Build history of the part. All positions in model axes, mm. Face numbers are marked on the shaded views. A direction names the side the tool comes from. Give positions to 0.01 mm unless a question says otherwise; leave off trailing zeros. Write each loop counter-clockwise with the first axis right and the second up, starting at its lowest first coordinate (ties: lowest second). Pieces come first, ordered by that corner, then holes. Notation, with made-up numbers: (-34, 54) -> (10, 54) arc R20 ccw to (10, 87) -> close; hole circle Ø7 at (1, 65.5). An arc over 180 degrees is marked (long way). Put each result on its own line as item: value. Start each with the question number.
Item 1: Drill centre lines: line 1 along Y through (x, z) = (0, -5.5); line 2 along Y through (x, z) = (10, -6.75); line 3 along Y through (x, z) = (-10, -10.25). Where is each one in solid material? Low to high.
Item 2: Slice it at B-B, the plane z = -1.25. Give the number of separate pieces and of enclosed holes in the cut face, plus the area to 3 significant figures.
Item 3: Tool access for the marked faces 1 and 2: list every direction of +Z, -Z, +X, -X, +Y, -Y with a clear straight run to the whole face (end or side of a thin tool).
Item 4: Flat gauge pins, fed straight in: pin 1 Ø3 at (x, z) = (-11.5, -2.5) entering from -Y; pin 2 Ø6 at (x, y) = (-2, 22) entering from +Z; pin 3 Ø5 at (y, z) = (22.5, -4) entering from -X. Where does each tip first touch, or does it go through?
Item 5: Slice it at A-A, the plane x = 0. List the corners of the cut face in (y, z), plus the area to 3 significant figures.
Item 6: Two-plate mould, pull along Y, no slides. Class the marked faces 3, 4 and 5: pulls with the +Y half, pulls with the -Y half, needs draft (parallel to the pull), parting line crosses it, or undercut.
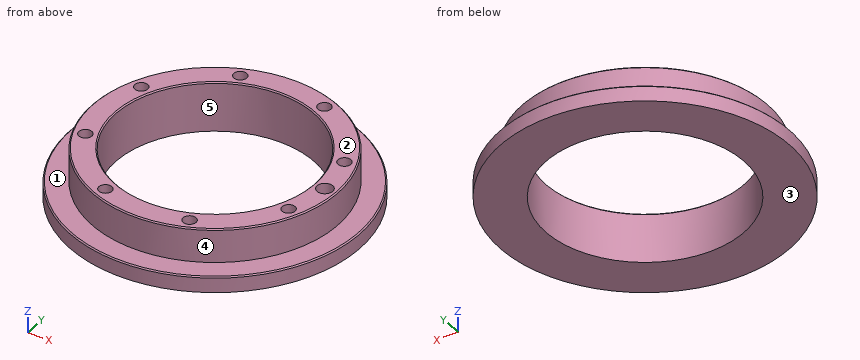
```python
from build123d import *

# Parameters (mm, degrees)
CHAMFER1_SIZE             = 0.3
F_4_000_X_6_0_DOWEL_D     = 4
F_4_000_X_6_0_DOWEL_DEPTH = 6
F_4_000_X_6_0_DOWEL_TIP   = 1.201721238
CIRPATTERN1_COUNT         = 8


with BuildPart() as part:
    # Sketch1 → Revolve1 (revolve)
    with BuildSketch(Plane(origin=(0, 0, 0), x_dir=(1, 0, 0), z_dir=(0, 1, 0))):
        Polygon((25, 0), (31, 0), (31, 8.5), (36.5, 8.5), (36.5, 12.5), (25, 12.5), align=None)
    revolve(axis=Axis((0, 0, 0), (0, 0, -1)))

    # Chamfer1
    chamfer1_edges = [part.edges().sort_by_distance(p)[0] for p in [
        (-36.5, 0, -8.5),
        (-25, 0, 0),
        (-31, 0, 0),
    ]]
    chamfer(chamfer1_edges, length=CHAMFER1_SIZE)

    # Ø4.000 x 6.0 Dowel
    with Locations(Plane.XY):
        with Locations((28, 0)):
            Hole(F_4_000_X_6_0_DOWEL_D / 2, depth=F_4_000_X_6_0_DOWEL_DEPTH)
            with Locations((0, 0, -(F_4_000_X_6_0_DOWEL_DEPTH + F_4_000_X_6_0_DOWEL_TIP / 2))):  # 118° drill point
                Cone(0, F_4_000_X_6_0_DOWEL_D / 2, F_4_000_X_6_0_DOWEL_TIP, mode=Mode.SUBTRACT)

    # Sketch5 → M4x0.7 x 6.0 Tapped Hole (revolve, cut)
    with BuildSketch(Plane(origin=(25.86862691, -10.715136106, 0), x_dir=(0, -1, 0), z_dir=(1, 0, 0))):
        Polygon((0, 0), (0, 12.491420021), (1.65, 11.5), (1.65, 0), align=None)
    m4x0_7_x_6_0_tapped_hole = revolve(axis=Axis((25.86862691, -10.715136106, 6.35), (0, 0, -1)), mode=Mode.SUBTRACT)

    # CirPattern1: M4x0.7 x 6.0 Tapped Hole ×8 about axis
    cirpattern1_axis = Axis((0, 0, 0), (0, 0, 1))
    for i in range(1, CIRPATTERN1_COUNT):
        add(m4x0_7_x_6_0_tapped_hole.rotate(cirpattern1_axis, i * 360 / CIRPATTERN1_COUNT), mode=Mode.SUBTRACT)


solid = part.part
```
Values follow:
1. line 1: -31 to -25, 25 to 31
1. line 2: -29.34 to -27.36, -24.38 to -22.91, 22.91 to 24.38, 27.36 to 29.34
1. line 3: -35.1 to -27.36, -24.38 to -22.91, 22.91 to 24.38, 27.36 to 35.1
2. separate pieces: 1
2. enclosed holes: 10
2. area: 975 mm2
3. face 1: +Z
3. face 2: +Z, +X, -X, +Y, -Y
4. pin 1: y = -29.34
4. pin 2: z = -0.21
4. pin 3: x = -23.69
5. outline: (-36.5, -12.5) -> (-25, -12.5) -> (-25, -0.3) -> (-25.3, 0) -> (-30.7, 0) -> (-31, -0.3) -> (-31, -8.5) -> (-36.2, -8.5) -> (-36.5, -8.8) -> close; (25, -12.5) -> (36.5, -12.5) -> (36.5, -8.8) -> (36.2, -8.5) -> (31, -8.5) -> (31, -0.3) -> (30.7, 0) -> (25.3, 0) -> (25, -0.3) -> close
5. area: 194 mm2
6. face 3: needs draft
6. face 4: parting line crosses it
6. face 5: undercut
